Build history of the part. All positions in model axes, mm. A direction names the side the tool comes from. Coordinates: 2 decimals unless noted, no trailing zeros. Write each loop counter-clockwise with the first axis right and the second up, starting at its lowest first coordinate (ties: lowest second). Pieces come first, ordered by that corner, then holes. Notation, with made-up numbers: (89, 28.5) -> (116, 28.5) arc R30 cw to (116, 50.5) -> close; hole circle Ø1 at (5, 89.25). An arc over 180 degrees is marked (long way). Write each question's results on one line, items separated by ' | '. Start each with the question number.
Q1. Drop flat-ended pins along their axis: pin 1 Ø3 at (x, z) = (39, -57.5) entering from +Y; pin 2 Ø3 at (x, z) = (9.5, -15.5) entering from +Y; pin 3 Ø3.5 at (x, z) = (43.72, -73.77) entering from -Y; pin 4 Ø0.6 at (x, z) = (1.5, -19) entering from +Y. Give the stop position or say it passes through.
Q2. Saw through at D-D on z = -56. Give the cut face in (x, y), and give its area (3 significant figures).
Q3. Drill centre lines: line 1 (Z direction, x = 8.8, y = 3.6); line 2 (X direction, y = 3.45, z = -15.1); line 3 (X direction, y = 16, z = -62.5). Where is each one in solid material? Low to high.
Q4. Saw through at C-C on x = 43.72. Give the cut face in (y, z), and give its area (3 significant figures).
Q5. Saw through at A-A on z = -86.5. Give the cut face in (x, y).
Q6. Two-plate mould, pull along X, no slides. Class faces 1 (the face through (1.01, 61.79, -10.12)), 2 (the face through (64, 33, -48)), 3 (the face through (62, 34, -48)): released by +X, released by -X, zero draft, split by the parting line, or undercut.
Q7. Tool access for faces 4 (the face through (28.317, 1.014, -75.615)), 5 (the face through (32, 2, -48)): list every direction of +Z, -Z, +X, -X, +Y, -Y with a clear straight run to the whole face (end or side of a thin tool).
Q8. Saw through at B-B on y = 9.5. Give the cut face in (x, z), and give its area (3 significant figures).
Autodesk Inventor part; units mm, degrees
ref_plane "YZ Plane" through (0, 0, 0) normal (1, 0, 0) x (0, 1, 0)
ref_plane "XZ Plane" through (0, 0, 0) normal (0, 1, 0) x (-1, 0, 0)
ref_plane "XY Plane" through (0, 0, 0) normal (0, 0, 1) x (1, 0, 0)
sketch "Sketch1" plane through (0, 0, 0) normal (0, 1, 0) x (-1, 0, 0)
  line L0 (0, 0) -> (-64, 0)
  line L1 (-64, 0) -> (-64, -97)
  line L2 (-64, -97) -> (0, -97)
  line L3 (0, -97) -> (0, 0)
  dimension "d1" = 64
  dimension "d2" = 97
extrude "Extrusion1" add sketch "Sketch1" along normal blind 60
shell "Shell1" thickness 2 removed faces 1 at (21.3333, 60, -64.6667)
sketch "Sketch2" plane through (2, 2, -2) normal (0, 1, 0) x (1, 0, 0)
  line L0 (60, 93) -> (0, 93)
  line L1 (30, 93) -> (30, 0) construction
  line L2 (60, 0) -> (0, 0)
  line L3 (0, 0) -> (0, 93)
  line L4 (0, 46.5) -> (60, 46.5) construction
  line L5 (60, 0) -> (60, 93)
  circle A0 centre (6.8, 79.9) radius 3
  circle A1 centre (6.8, 79.9) radius 1.75
  circle A2 centre (53.2, 79.9) radius 3
  circle A3 centre (53.2, 79.9) radius 1.75
  circle A4 centre (6.8, 13.1) radius 3
  circle A5 centre (6.8, 13.1) radius 1.75
  circle A6 centre (53.2, 13.1) radius 3
  circle A7 centre (53.2, 13.1) radius 1.75
  point P0 (-2, -2)
  dimension "d6" = 6
  dimension "d7" = 1.25
  dimension "d8" = 23.2
  dimension "d9" = 33.4
extrude "Extrusion2" add sketch "Sketch2" along normal blind 6 contours A0 | A2 | A4 | A6
sketch "Sketch3" plane through (2, 2, -2) normal (0, 1, 0) x (1, 0, 0)
  circle A0 centre (53.2, 79.9) radius 1.75
  circle A1 centre (27, 68.41) radius 5.25
  circle A2 centre (41.72, 71.77) radius 2.75
  circle A3 centre (49.23, 71.77) radius 2.75
  point P0 (-2, -2)
  dimension "d12" = 11.49
  dimension "d13" = 26.2
  dimension "d14" = 10.5
  dimension "d15" = 0
  dimension "d16" = 5.5
  dimension "d17" = 5.5
  dimension "d18" = 3.97
  dimension "d19" = 8.13
  dimension "d20" = 7.51
extrude "Extrusion3" cut sketch "Sketch3" against normal through all contours A1 | A2 | A3
sketch "Sketch4" plane through (64, 0, 0) normal (1, 0, 0) x (0, 0, -1)
  line L0 (0, 0) -> (97, 0)
  line L1 (48.5, 0) -> (48.5, 60) construction
  line L2 (95, 60) -> (2, 60)
  line L3 (4, 60) -> (17, 60)
  line L4 (14, 67) -> (7, 67)
  line L5 (0, 0) -> (0, 60)
  line L6 (4, 60) -> (7, 67)
  line L7 (17, 60) -> (14, 67)
  circle A0 centre (10.5, 63.5) radius 1.75
  line L8 (83, 67) -> (90, 67)
  line L9 (93, 60) -> (90, 67)
  line L10 (80, 60) -> (83, 67)
  circle A1 centre (86.5, 63.5) radius 1.75
  line L11 (80, 60) -> (93, 60)
  dimension "d28" = 7
  dimension "d29" = 4
  dimension "d30" = 13
  dimension "d31" = 7
  dimension "d32" = 3
  dimension "d33" = 3.5
  dimension "d34" = 3.5
  dimension "d35" = 6.5
extrude "Extrusion4" add sketch "Sketch4" against normal blind 64
sketch "Sketch5" plane through (0, 60, 0) normal (0, 1, 0) x (1, 0, 0)
  line L0 (62, 2) -> (2, 2)
  line L1 (2, 93) -> (2, 95)
  line L2 (62, 2) -> (2, 2)
  line L3 (2, 2) -> (2, 95)
  line L4 (2, 95) -> (62, 95)
  line L5 (62, 95) -> (62, 2)
  point P0 (0, 0)
extrude "Extrusion5" cut sketch "Sketch5" along normal through all
sketch "Sketch6" plane through (0, 0, -97) normal (-1, 0, 0) x (0, 0, 1)
  line L0 (2, 2) -> (2, 60)
  line L1 (17, 60) -> (80, 60)
  line L2 (85.5, 49.8) -> (73.5, 49.8)
  line L3 (73.5, 49.8) -> (73.5, 42.3)
  line L4 (73.5, 42.3) -> (85.5, 42.3)
  line L5 (85.5, 42.3) -> (85.5, 49.8)
  line L6 (97, 0) -> (97, 60)
  dimension "d48" = 7.5
  dimension "d49" = 10.2
  dimension "d51" = 11.5
  dimension "d52" = 23.5
extrude "Extrusion6" cut sketch "Sketch6" against normal up to next
properties part number "Housing for Filter"
Returned:
1) pin 1: stops at y = 2 | pin 2: stops at y = 8 | pin 3: passes through | pin 4: stops at y = 60
2) outline: (0, 0) -> (64, 0) -> (64, 60) -> (62, 60) -> (62, 2) -> (2, 2) -> (2, 60) -> (0, 60) -> close | area: 360 mm2
3) line 1: z = -97 to -95, -84.9 to -83.65, -80.15 to -78.9, -18.1 to -16.85, -13.35 to -12.1, -2 to 0 | line 2: x = 0 to 2, 5.8 to 7.05, 10.55 to 11.8, 52.2 to 53.45, 56.95 to 58.2, 62 to 64 | line 3: x = 0 to 2, 62 to 64
4) outline: (0, -97) -> (60, -97) -> (60, -95) -> (2, -95) -> (2, -76.52) -> (0, -76.52) -> close; (0, -71.02) -> (2, -71.02) -> (2, -2) -> (60, -2) -> (60, 0) -> (0, 0) -> close | area: 415 mm2
5) outline: (0, 0) -> (64, 0) -> (64, 61.75) -> (62, 61.75) -> (62, 2) -> (2, 2) -> (2, 61.75) -> (0, 61.75) -> close; (0, 65.25) -> (2, 65.25) -> (2, 67) -> (0, 67) -> close; (62, 65.25) -> (64, 65.25) -> (64, 67) -> (62, 67) -> close
6) face 1: zero draft | face 2: released by +X | face 3: undercut
7) face 4: +Y, -Y | face 5: +Y
8) outline: (0, -97) -> (64, -97) -> (64, 0) -> (0, 0) -> close; hole (2, -95) -> (62, -95) -> (62, -2) -> (2, -2) -> close | area: 628 mm2
